Read the model definition and answer for the solid it produces. Units are mm, in the model's axes. A direction names the side the tool comes from. Coordinates: 2 decimals unless noted, no trailing zeros. Order: outer loops, then holes, each group sorted by start corner. A loop starts at its lowest first (then second) coordinate and runs counter-clockwise, first axis right, second up. Notation, with made-up numbers: (18, 51) -> (22, 51) arc R19 cw to (22, 57) -> close; hole circle Ø6 at (77, 33). An arc over 180 degrees is marked (long way). Use CSV: the item, a comma, the result in double quotes.
```python
from build123d import *

# Parameters (mm, degrees)
F0_W     = 180.109705776
F0_H     = 138.2466368377
F1_DEPTH = 101.6
F2_W     = 161.1165106297
F2_H     = 112.253382802
F3_DEPTH = 88.9
F4_R     = 12.7
F5_DEPTH = 9.0965814888


with BuildPart() as f1:
    # F0 (on Top) → F1 (new body)
    with BuildSketch(Plane.XY):
        with Locations((-28.1288344413, 0.5972143263)):
            Rectangle(F0_W, F0_H)
    extrude(amount=F1_DEPTH)

    # F2 (on face) → F3 (cut)
    with BuildSketch(Plane.XY.offset(101.6)):
        with Locations((-27.728818357, 1.6608275473)):
            Rectangle(F2_W, F2_H)
    extrude(amount=-F3_DEPTH, mode=Mode.SUBTRACT)

    # F4 (on face) → F5 (cut, through all)
    with BuildSketch(Plane.YZ.offset(61.9260184467)):
        with Locations((0.5972143263, 50.8)):
            Circle(F4_R)
    extrude(amount=-F5_DEPTH, mode=Mode.SUBTRACT)


solid = f1.part
```
Item 1: The mould has two halves that part along Y. Classify faces 1 (the flat face through (-42, -55, 101.6)), 2 (the cylindrical face through (57.441, 6.457, 39.533)), 3 (the flat face through (-29, -68.526, 50)): +Y half, -Y half, draft (parallel to the pull), parting line (faces both ways), or undercut.
Return value:
face 1,"draft"
face 2,"undercut"
face 3,"-Y half"
Item 2: This flat-tipped pin is pushed along its axis until it touches: P1, Ø2, axis at x = 42.5, y = 26, coming from the +Z side. Where does it stop, or does it pass through?
Return value:
P1,"stops at z = 12.7"
Item 3: Find section D-D, the plane z = 50.8. Give the vertices of the cut face in (x, y).
Return value:
outline,"(-118.18, -68.53) -> (61.93, -68.53) -> (61.93, -12.1) -> (52.83, -12.1) -> (52.83, -54.47) -> (-108.29, -54.47) -> (-108.29, 57.79) -> (52.83, 57.79) -> (52.83, 13.3) -> (61.93, 13.3) -> (61.93, 69.72) -> (-118.18, 69.72) -> close"
Item 4: A tool of negligible diameter and unlimited length cuts with its end or side. For faces 4 (the flat face through (-29, 57.788, 58)), 5 (the flat face through (-29, 2, 0)), from which of +Z, -Z, +X, -X, +Y, -Y can it reach the whole face along a straight path? Write none if from no direction.
Return value:
face 4,"+Z"
face 5,"-Z, +X, -X, +Y, -Y"
Item 5: Find section A-A, the plane z = 89.5. Give the vertices of the cut face in (x, y), then the cut area to 3 significant figures.
Return value:
outline,"(-118.18, -68.53) -> (61.93, -68.53) -> (61.93, 69.72) -> (-118.18, 69.72) -> close; hole (-108.29, -54.47) -> (52.83, -54.47) -> (52.83, 57.79) -> (-108.29, 57.79) -> close"
area,"6,810 mm^2"
Item 6: Find section C-C, the plane y = 3.5. Give the vertices of the cut face in (x, z).
Return value:
outline,"(-118.18, 0) -> (61.93, 0) -> (61.93, 38.44) -> (52.83, 38.44) -> (52.83, 12.7) -> (-108.29, 12.7) -> (-108.29, 101.6) -> (-118.18, 101.6) -> close; (52.83, 63.16) -> (61.93, 63.16) -> (61.93, 101.6) -> (52.83, 101.6) -> close"
Item 7: Straight lines are drawn through the part: line 1 along Y through (x, z) = (-98.5, 15.5); line 2 along X through (y, z) = (-26.5, 72.5); line 3 along Y through (x, z) = (59, 50). For each, find the intervals that lie inside material, in ascending order.
Return value:
line 1,"y = -68.53 to -54.47, 57.79 to 69.72"
line 2,"x = -118.18 to -108.29, 52.83 to 61.93"
line 3,"y = -68.53 to -12.08, 13.27 to 69.72"
Item 8: Find section B-B, the plane y = 49. Give the vertices of the cut face in (x, z).
Return value:
outline,"(-118.18, 0) -> (61.93, 0) -> (61.93, 101.6) -> (52.83, 101.6) -> (52.83, 12.7) -> (-108.29, 12.7) -> (-108.29, 101.6) -> (-118.18, 101.6) -> close"
